Part model, mm, in its own coordinate system. Face numbers are marked on the shaded views. A direction names the side the tool comes from. Coordinates: 2 decimals unless noted, no trailing zeros. Loops run counter-clockwise (first coordinate to the right, second up) from the corner with the lowest first, then second, coordinate; pieces in that order, holes last.
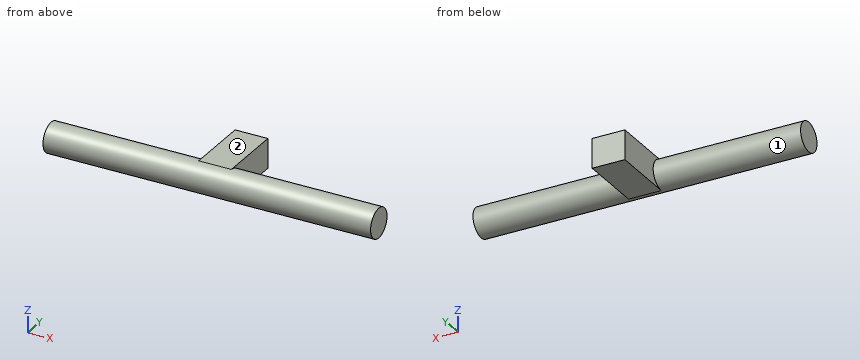
```python
from build123d import *

# Parameters (mm, degrees)
ESQUISSE1_R        = 45
BOSS_EXTRU_1_DEPTH = 500
ESQUISSE2_W        = 90
ESQUISSE2_H        = 200
BOSS_EXTRU_2_DEPTH = 50


with BuildPart() as part:
    # Esquisse1 → Boss.-Extru.1 (new body, symmetric)
    with BuildSketch(Plane(origin=(0, 0, 0), x_dir=(0, 0, -1), z_dir=(1, 0, 0))):
        Circle(ESQUISSE1_R)
    extrude(amount=BOSS_EXTRU_1_DEPTH, both=True)

    # Esquisse2 → Boss.-Extru.2 (add, symmetric)
    with BuildSketch(Plane(origin=(0, 0, 0), x_dir=(0, 0, -1), z_dir=(1, 0, 0))):
        with Locations((0, 100)):
            Rectangle(ESQUISSE2_W, ESQUISSE2_H)
    extrude(amount=BOSS_EXTRU_2_DEPTH, both=True)


solid = part.part
```
Q1. Drop flat-ended pins along their axis: P1, Ø10, axis at y = 47.5, z = -5, coming from the -X side; P2, Ø1.5, axis at x = -297, y = 25.5, coming from the -Z side; P3, Ø5, axis at x = -164, y = 36.5, coming from the +Z side; P4, Ø1.5, axis at y = 61.5, z = 29.5, coming from the +X side. Give the stop position or say it passes through.
Q2. Saw through at B-B (y = 145). List the corners of the cut face in (x, z).
Q3. Tool access for the marked faces 1 and 2: list every direction of +Z, -Z, +X, -X, +Y, -Y with a clear straight run to the whole face (end or side of a thin tool).
Q4. Saw through at A-A (z = 0). List the corners of the cut face in (x, y).
Q5. Probe line 1 (X direction, y = 169.5, z = -33); line 2 (Y direction, x = 277.5, z = -2); line 3 (Y direction, x = -316, z = 8). List the from-to ranges inside material, lowest first.
Q6. Saw through at D-D (x = -329). List the corners of the cut face in (y, z).
Q7. Saw through at C-C (x = 19.5). List the corners of the cut face in (y, z).
Checked values:
1. P1: stops at x = -500
1. P2: stops at z = -37.58
1. P3: stops at z = 29.48
1. P4: stops at x = 50
2. outline: (-50, -45) - (50, -45) - (50, 45) - (-50, 45) - close
3. face 1: none
3. face 2: +Z, +X, -X, +Y, -Y
4. outline: (-500, -45) - (500, -45) - (500, 45) - (50, 45) - (50, 200) - (-50, 200) - (-50, 45) - (-500, 45) - close
5. line 1: x = -50 to 50
5. line 2: y = -44.96 to 44.96
5. line 3: y = -44.28 to 44.28
6. outline: circle Ø90 at (0, 0)
7. outline: (0, -45) - (200, -45) - (200, 45) - (0, 45) arc R45 ccw to start
